Check sheet for the modelled part. Datum: model origin and axes. Units: mm. A direction names the side the tool comes from. Round coordinates to 2 decimals unless told otherwise and drop trailing zeros. Loops run counter-clockwise (first coordinate to the right, second up) from the corner with the lowest first, then second, coordinate; pieces in that order, holes last. Notation, with made-up numbers: M 9.5,41 L 64.5,41 A10 cw 64.5,59 Z; hole C -31.5,-23 d11. An arc over 180 degrees is marked long. One line per question, with ' | ' between items. Start each with the question number.
(1) Tool access check on faces 1 (the face through (-4, 9, 0)), 2 (the face through (1, 9, 10)), 3 (the face through (1, 15.575, 9)). Record the directions out of +Z, -Z, +X, -X, +Y, -Y that give a thin tool (end or side, any length) a straight path to the whole face; none if there is none.
(2) Draft check along X on faces 4 (the face through (7.496, 9, 5)), 5 (the face through (6, 9, 0)), 6 (the face through (1, 22.425, 9)). Enter one of: +X half, -X half, draft (parallel to the pull), parting line (faces both ways), or undercut.
(3) Section check C-C (y = 17.5). Record the boundary of the cut face in (x, z), and give its area (3 significant figures).
(4) Thickness scan on probe 1 along Y at (x, z) = (2, 8) (3 decimals); probe 2 along X at (y, z) = (-1, 1.25); probe 3 along Y at (x, z) = (3.5, 7.25). Record the ranges inside material, lowest first. Write a range as [from, to].
(5) Section check A-A (x = 2.75). Record the boundary of the cut face in (y, z) (3 decimals), and give its area (3 significant figures).
(6) Section check D-D (x = -2). Record the boundary of the cut face in (y, z).
(7) Section check B-B (z = 7.5). Record the boundary of the cut face in (x, y) (3 decimals).
(8) Go/stop test with flat-tipped pins: P1, Ø1, axis at x = 7, y = 6.5, coming from the -Z side; P2, Ø3.5, axis at x = 1.5, y = 0, coming from the +Z side; P3, Ø3.5, axis at x = 1.25, y = 19, coming from the -Z side; P4, Ø3, axis at x = -1, y = 14.5, coming from the -Z side. Record where each tip stops, or that it passes through.
```python
from build123d import *

# Parameters (mm, degrees)
BOSS_EXTRUDE1_DEPTH      = 25
BOSS_EXTRUDE1_DEPTH_BACK = 7
SKETCH3_R                = 2
CUT_EXTRUDE1_DEPTH       = 25
CUT_EXTRUDE2_DEPTH       = 3


with BuildPart() as part:
    # Sketch2 → Boss-Extrude1 (new body, two sides)
    with BuildSketch(Plane(origin=(0, 0, 0), x_dir=(1, 0, 0), z_dir=(0, 1, 0))) as boss_extrude1_sk:
        Polygon((-4.989079304, 0), (-2.989079304, 0), (1.253561383, 4.242640687), (5.49620207, 0), (7.49620207, 0), (7.49620207, -10), (-4.989079304, -10), align=None)
    extrude(amount=BOSS_EXTRUDE1_DEPTH)
    extrude(boss_extrude1_sk.sketch, amount=-BOSS_EXTRUDE1_DEPTH_BACK)

    # Sketch3 → Cut-Extrude1 (cut)
    with BuildSketch(Plane.XY.offset(10)):
        with Locations((1.253561383, 19)):
            Circle(SKETCH3_R)
        with Locations((1.253561383, -1)):
            Circle(SKETCH3_R)
    extrude(amount=-CUT_EXTRUDE1_DEPTH, mode=Mode.SUBTRACT)

    # Sketch4 → Cut-Extrude2 (cut)
    with BuildSketch(Plane.XY.offset(10)):
        Polygon((5.208410727, -1), (3.230986055, 2.425), (-0.723863289, 2.425), (-2.701287961, -1), (-0.723863289, -4.425), (3.230986055, -4.425), align=None)
        Polygon((3.230986055, 22.425), (5.208410727, 19), (3.230986055, 15.575), (-0.723863289, 15.575), (-2.701287961, 19), (-0.723863289, 22.425), align=None)
    extrude(amount=-CUT_EXTRUDE2_DEPTH, mode=Mode.SUBTRACT)


solid = part.part
```
The answers:
1) face 1: -Z, -X, +Y, -Y | face 2: +Z, +X, -X, +Y, -Y | face 3: +Z
2) face 4: +X half | face 5: draft | face 6: undercut
3) outline: M -4.99,0 L -2.99,0 L -0.07,-2.92 L -0.07,7 L -1.84,7 L -1.84,10 L -4.99,10 Z; M 2.58,-2.92 L 5.5,0 L 7.5,0 L 7.5,10 L 4.34,10 L 4.34,7 L 2.58,7 Z | area: 96.3 mm²
4) probe 1: [-7, -4.425], [2.425, 15.575], [22.425, 25] | probe 2: [-4.99, -0.75], [3.25, 7.5] | probe 3: [-7, -3.96], [1.96, 16.04], [21.96, 25]
5) outline: M -7,-2.746 L -2.327,-2.746 L -2.327,7 L -4.425,7 L -4.425,10 L -7,10 Z; M 0.327,-2.746 L 17.673,-2.746 L 17.673,7 L 15.575,7 L 15.575,10 L 2.425,10 L 2.425,7 L 0.327,7 Z; M 20.327,-2.746 L 25,-2.746 L 25,10 L 22.425,10 L 22.425,7 L 20.327,7 Z | area: 315 mm²
6) outline: M -7,-0.99 L 25,-0.99 L 25,10 L 20.21,10 L 20.21,7 L 17.79,7 L 17.79,10 L 0.21,10 L 0.21,7 L -2.21,7 L -2.21,10 L -7,10 Z
7) outline: M -4.989,-7 L 7.496,-7 L 7.496,25 L -4.989,25 Z; hole M -2.701,-1 L -0.724,-4.425 L 3.231,-4.425 L 5.208,-1 L 3.231,2.425 L -0.724,2.425 Z; hole M -2.701,19 L -0.724,15.575 L 3.231,15.575 L 5.208,19 L 3.231,22.425 L -0.724,22.425 Z
8) P1: z = 0 | P2: z = 7 | P3: through | P4: z = -3.49
